```python
from build123d import *

# Parameters (mm, degrees)
F0_W     = 20
F0_H     = 5
F1_DEPTH = 5
F2_SIZE2 = 4.99999
F2_SIZE  = 19.09999


# Not quite as in the source:
# - a fillet or chamfer is up to 0.001 mm smaller than in the source, because OpenCascade refuses the exact size


with BuildPart() as f1:
    # F0 (on Top) → F1 (new body)
    with BuildSketch(Plane.XY):
        Rectangle(F0_W, F0_H)
    extrude(amount=F1_DEPTH)

    # F2 (size 19.1 and 5 in the source; OpenCascade refuses exactly that, so slightly less here)
    f2_edges = [f1.edges().sort_by_distance(p)[0] for p in [
        (10, 0, 5),
    ]]
    f2_side = f1.faces().sort_by_distance((0, 0, 5))[0]
    chamfer(f2_edges, length=F2_SIZE, length2=F2_SIZE2, reference=f2_side)


solid = f1.part
```
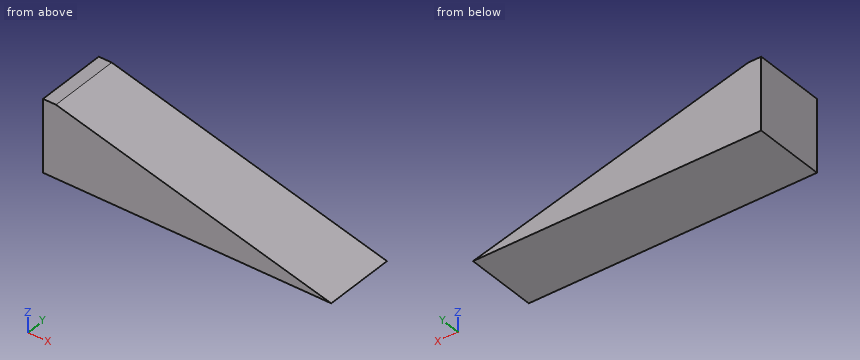
Model file for the job. Use its own axes, mm. Coordinates: 2 decimals unless noted, no trailing zeros. Loops run counter-clockwise (first coordinate to the right, second up) from the corner with the lowest first, then second, coordinate; pieces in that order, holes last. Notation, with made-up numbers: (24, 13) - (82, 13) arc R20 cw to (82, 43) - close; hole circle Ø4 at (59, 47.25). An arc over 180 degrees is marked (long way). Answer as a JSON object with one key per item and string values. Group by question number.
(1) Cut at C-C (z = 3.45). Give the cut face in (x, y).
(2) Probe line 1 along Z through (x, y) = (-3.5, -1.15); line 2 along Z through (x, y) = (-8.5, -2.1). List the from-to ranges inside material, lowest first.
(3) Cut at B-B (x = 0). Give the cut face in (y, z).
(4) Flat gauge pin, fed straight in: pin 1 (1.5 mm diameter, centred on x = 2, y = -0.5, fed in from -Z). Where does the tip first touch, or does it go through?
Geometry says:
{
 "1": {"outline": "(-10, -2.5) - (-3.18, -2.5) - (-3.18, 2.5) - (-10, 2.5) - close"},
 "2": {"line 1": "z = 0 to 3.53", "line 2": "z = 0 to 4.84"},
 "3": {"outline": "(-2.5, 0) - (2.5, 0) - (2.5, 2.62) - (-2.5, 2.62) - close"},
 "4": {"pin 1": "stops at z = 0"}
}
